Autodesk Fusion 360 part; units mm, degrees
sketch "Sketch1" plane through (0, 0, 0) normal (0, 1, 0) x (1, 0, 0)
  circle A0 centre (0, 0) radius 20
  dimension "d1" = 40
extrude "Extrude1" add sketch "Sketch1" along normal blind 140
sketch "Sketch2" plane through (0, 140, 0) normal (0, 1, 0) x (-1, 0, 0)
  circle A0 centre (0, 0) radius 20
  circle A1 centre (0, 0) radius 17
  dimension "d4" = 34
extrude "Extrude2" add sketch "Sketch2" along normal blind 20 contours A1
sketch "Sketch3" plane through (0, 0, 0) normal (1, 0, 0) x (0, 0, -1)
sketch "Sketch4" plane through (0, 0, 0) normal (0, -1, 0) x (1, 0, 0)
  circle A0 centre (0, 0) radius 20
  line L0 (0, 20) -> (-20, 20)
  line L1 (-20, 20) -> (-20, 10)
  line L2 (-20, 10) -> (20, 10)
  line L3 (20, 10) -> (20, 20)
  line L4 (20, 20) -> (0, 20)
extrude "Extrude3" add sketch "Sketch4" against normal blind 40 contours A0 L2 L3 L4 | A0 L0 L1 L2
sketch "Sketch5" plane through (20, 0, 0) normal (1, 0, 0) x (0, 0, -1)
  line L0 (-20, 0) -> (-10, 0)
  line L1 (-10, 0) -> (-10, 40)
  line L2 (-10, 40) -> (-20, 40)
  line L3 (-20, 40) -> (-20, 0)
sketch "Sketch6" plane through (0, 0, 0) normal (0, 1, 0) x (1, 0, 0)
extrude "Extrude4" add 1 faces at (0, 13.3333, 20) along direction (0, 0, 1) blind 5
sketch "Sketch7" plane through (0, 0, 0) normal (0, 1, 0) x (1, 0, 0)
  circle A0 centre (0, 0) radius 20.3
  dimension "d15" = 40.6
extrude "Extrude5" cut sketch "Sketch7" along normal blind 165
extrude "Extrude6" cut 1 faces at (-20, 13.3333, 20) along direction (1, 0, 0) blind 3
extrude "Extrude7" cut 1 faces at (20, 13.3333, 20) along direction (-1, 0, 0) blind 3
sketch "Sketch8" plane through (0, 0, 0) normal (1, 0, 0) x (0, 0, -1)
  line L0 (-11.0946, 40) -> (-14.0946, 40)
  line L1 (-14.0946, 40) -> (-14.0946, -0.0914)
  line L2 (-14.0946, -0.0914) -> (-11.0946, -0.0914)
  line L3 (-11.0946, -0.0914) -> (-11.0946, 40)
  point P0 (-11.0946, 40)
  dimension "d22" = 3
extrude "Extrude8" cut sketch "Sketch8" along normal blind 20 and the other way blind 20
Geometry: final body of the model. Coordinates: model frame, mm. Coordinates: 2 decimals unless noted, no trailing zeros. Loops run counter-clockwise (first coordinate to the right, second up) from the corner with the lowest first, then second, coordinate; pieces in that order, holes last. Notation, with made-up numbers: (-14, 23.5) - (4, 23.5) arc R23 ccw to (4, 55.5) - close; hole circle Ø3 at (81, 65.25). An arc over 180 degrees is marked (long way). One line per question, with ' | ' between items. Start each with the question number.
(1) Cut plane D-D on x = 13. Output: boundary loops of the cut face in (y, z).
(2) Cut plane C-C on z = 19.5. Output: boundary loops of the cut face in (x, y).
(3) Cut plane B-B on y = 36. Output: boundary loops of the cut face in (x, z).
(4) First-contact query: pin 1 (2 mm diameter, centred on x = -2, y = 19.5, fed in from -Z). Flat tip, straight axial feed; report the tip coordinate or a pass-through.
(5) Ray query, L1, parallel to Z at x = 0, y = 19.5; L2, parallel to X at y = 30, z = 16.75; L3, parallel to X at y = 38, z = 18.25. Return the intervals inside material, ascending. Write a range as from..to.
(6) Cut plane A-A on z = 16. Output: boundary loops of the cut face in (x, y), and give its area (3 significant figures).
(7) Draft query along X for faces 1 (the cylindrical face through (0.2, 19.7, 20.3)), 2 (the flat face through (17, 20, 19)), 3 (the flat face through (16, 20, 14.095)). Return one class per face: +X half, -X half, draft (parallel to the pull), parting line (faces both ways), or undercut.
Here are the results:
1) outline: (0, 15.59) - (40, 15.59) - (40, 25) - (0, 25) - close
2) outline: (-17, 0) - (-5.64, 0) - (-5.64, 40) - (-17, 40) - close; (5.64, 0) - (17, 0) - (17, 40) - (5.64, 40) - close
3) outline: (-17, 14.09) - (-14.61, 14.09) arc R20.3 cw to (14.61, 14.09) - (17, 14.09) - (17, 25) - (-17, 25) - close
4) pin 1: z = 20.08
5) L1: 20.3..25 | L2: -17..-11.47, 11.47..17 | L3: -17..-8.89, 8.89..17
6) outline: (-17, 0) - (-12.49, 0) - (-12.49, 40) - (-17, 40) - close; (12.49, 0) - (17, 0) - (17, 40) - (12.49, 40) - close | area: 361 mm²
7) face 1: undercut | face 2: +X half | face 3: draft
